from build123d import *

# Parameters (mm, degrees)
F0_R     = 1.25
F1_DEPTH = 26
F2_R     = 1.25
F3_DEPTH = 25
F4_DEPTH = 16.5
F5_W     = 5
F5_H     = 10
F6_DEPTH = 14
F7_R     = 1
F8_R     = 0.5


with BuildPart() as f1:
    # F0 (on Front) → F1 (new body)
    with BuildSketch(Plane.XZ):
        Polygon((-63.544681223, 48.3711008589), (-70.961089088, 25.5457444679), (-4.4139098395, 3.8321440613), (3.0292749177, 26.7399112527), align=None)
        with Locations((-7.6221936302, 10.1384017438)):
            Circle(F0_R, mode=Mode.SUBTRACT)
        with Locations((-3.2710926357, 23.5297136431)):
            Circle(F0_R, mode=Mode.SUBTRACT)
        with Locations((-64.662632986, 28.7500592351)):
            Circle(F0_R, mode=Mode.SUBTRACT)
        with Locations((-60.3344836134, 42.0707333056)):
            Circle(F0_R, mode=Mode.SUBTRACT)
    extrude(amount=F1_DEPTH)

    # F2 (on face) → F3 (cut)
    with BuildSketch(Plane(origin=(0.7053652428, 0, 2.1617818497), x_dir=(0.9506732609, 0, -0.3101940539), z_dir=(-0.3101940539, 0, -0.9506732609))):
        with Locations((-65.1349479941, 18)):
            Circle(F2_R)
        with Locations((-65.1348943617, 8)):
            Circle(F2_R)
        with Locations((-15.6349479941, 18)):
            Circle(F2_R)
        with Locations((-15.6348943617, 8)):
            Circle(F2_R)
    extrude(amount=-F3_DEPTH, mode=Mode.SUBTRACT)

    # F2 (on face) → F4 (cut)
    with BuildSketch(Plane(origin=(0.7053652428, 0, 2.1617818497), x_dir=(0.9506732609, 0, -0.3101940539), z_dir=(-0.3101940539, 0, -0.9506732609))):
        Polygon((-19.3849479941, 23.5), (-61.3849479941, 23.5), (-61.3849479941, 15.5), (-64.3849479941, 15.5), (-64.3849479941, 10.5), (-61.3849479941, 10.5), (-61.3849479941, 2.5), (-19.3849479941, 2.5), align=None)
    extrude(amount=-F4_DEPTH, mode=Mode.SUBTRACT)

    # F5 (on face) → F6 (cut)
    with BuildSketch(Plane(origin=(-71.6926139783, 0, 23.294342356), x_dir=(0, -1, 0), z_dir=(-0.9510565163, 0, 0.3090169944))):
        with Locations((13, 13.8672642722)):
            Rectangle(F5_W, F5_H)
    extrude(amount=-F6_DEPTH, mode=Mode.SUBTRACT)

    # F7 (call 1 of 4: OpenCascade refuses the feature's edges together)
    f7_edges = [f1.edges().sort_by_distance(p)[0] for p in [
        (-67.407394, -10.5, 36.482894),
        (-67.407394, -15.5, 36.482894),
        (-65.862309, -13, 41.238177),
        (-68.952479, -13, 31.727612),
    ]]
    fillet(f7_edges, radius=F7_R)

    # F7#2 (call 2 of 4)
    f7_2_edges = [f1.edges().sort_by_distance(p)[0] for p in [
        (-55.092562, -15.5, 29.046082),
    ]]
    fillet(f7_2_edges, radius=F7_R)

    # F7#3 (call 3 of 4)
    f7_3_edges = [f1.edges().sort_by_distance(p)[0] for p in [
        (-55.092562, -10.5, 29.046082),
    ]]
    fillet(f7_3_edges, radius=F7_R)

    # F7#4 (call 4 of 4)
    f7_4_edges = [f1.edges().sort_by_distance(p)[0] for p in [
        (-58.483196, -13, 28.325936),
    ]]
    fillet(f7_4_edges, radius=F7_R)

    # F8
    f8_edges = [f1.edges().sort_by_distance(p)[0] for p in [
        (-57.651663, -20, 21.203028),
        (-60.503683, -13, 22.13361),
        (-59.55301, -10.5, 21.823416),
        (-57.930109, -10.207107, 21.293881),
        (-37.687525, -23.5, 14.688953),
        (-55.092562, -23.5, 29.046082),
        (-52.533462, -20, 36.889137),
        (-32.569323, -23.5, 30.375061),
        (-52.533462, -6, 36.889137),
        (-55.092562, -2.5, 29.046082),
        (-32.569323, -2.5, 30.375061),
        (-37.687525, -2.5, 14.688953),
        (-15.164286, -2.5, 16.017932),
        (-15.164286, -23.5, 16.017932),
        (-17.723386, -13, 8.174877),
        (-12.605185, -13, 23.860986),
        (-57.651663, -6, 21.203028),
        (-70.961089, -13, 25.545744),
        (-4.41391, -13, 3.832144),
        (3.029275, -13, 26.739911),
        (-63.544681, -13, 48.371101),
    ]]
    fillet(f8_edges, radius=F8_R)


solid = f1.part
Build history of the part. All positions in model axes, mm. A direction names the side the tool comes from. Give positions to 0.01 mm unless a question says otherwise; leave off trailing zeros. Put each result on its own line as item: value.
Item 1: Flat gauge pins, fed straight in: pin 1 Ø12 at (y, z) = (-12, 35) entering from -X; pin 2 Ø13.5 at (x, z) = (-30.5, 21.5) entering from +Y; pin 3 Ø1.5 at (y, z) = (-18, 19.5) entering from +X; pin 4 Ø8 at (x, y) = (-42, -11.5) entering from -Z. Where does each tip first touch, or does it go through?
From the geometry:
pin 1: stops at x = -69.84
pin 2: stops at y = 0
pin 3: stops at x = 0.92
pin 4: stops at z = 32.15
Item 2: Probe line 1 (Y direction, x = -16.5, z = 18.5); line 2 (Y direction, x = -63.5, z = 33); line 3 (Z direction, x = -8, y = -5.25). List the from-to ranges inside material, lowest first. Write a range as [from, to].
From the geometry:
line 1: y = [-26, -23.5], [-2.5, 0]
line 2: y = [-26, -15.5], [-10.5, 0]
line 3: z = [5, 8.95], [11.33, 30.32]
Item 3: 3-axis set-ups, long thin cutter, end or side, ignore diameter. For faces 4 (the cylindrical face through (-6.95, -12.82, 11.19)), 5 (the flat face through (-61, -15.5, 33)), 6 (the flat face through (-59.58, -13.04, 24.96)): which of +Z, -Z, +X, -X, +Y, -Y reach the whole face in a straight line?
From the geometry:
face 4: +Y, -Y
face 5: none
face 6: -Z
Item 4: Two-plate mould, pull along X, no slides. Class faces 1 (the cylindrical face through (-54.92, -23.35, 29.11)), 2 (the cylindrical face through (-67.1, -10.2, 36.5)), 3 (the flat face through (-0.742, -12.818, 15.133)): +X half, -X half, draft (parallel to the pull), parting line (faces both ways), or undercut.
From the geometry:
face 1: undercut
face 2: -X half
face 3: +X half
Item 5: Slice it at A-A, the plane y = -12. Give the number of separate pieces and of enclosed holes in the cut face, plus the area to 3 significant figures.
From the geometry:
separate pieces: 2
enclosed holes: 4
area: 810 mm2
